The model under review builds one solid part; all positions refer to its coordinate system, in mm. A direction names the side the tool comes from. Give positions to 0.01 mm unless a question says otherwise; leave off trailing zeros. Write each loop counter-clockwise with the first axis right and the second up, starting at its lowest first coordinate (ties: lowest second). Pieces come first, ordered by that corner, then holes.
from build123d import *

# Parameters (mm, degrees)
SM_BASE_FLANGE_1_DEPTH = 2066
CUT_EXTRUDE_2_DEPTH    = 2.3
CUT_EXTRUDE_3_REACH    = 2082.296
CUT_EXTRUDE_4_REACH    = 2082.367
SKETCH_8_R             = 7


# Sheet-metal steps are written as plain solids
with BuildPart() as part:
    # Sketch 1 → Sm Base Flange 1 (new body)
    with BuildSketch(Plane.XY):
        with BuildLine():
            Line((33, 0), (3.3, 0))
            ThreePointArc((3.3, 0), (0.966547622, 0.966547622), (0, 3.3))
            Line((0, 3.3), (0, 52))
            ThreePointArc((0, 52), (0.966547622, 54.333452378), (3.3, 55.3))
            Line((3.3, 55.3), (22.085786438, 55.3))
            ThreePointArc((22.085786438, 55.3), (22.46846987, 55.376120467), (22.792893219, 55.592893219))
            Line((22.792893219, 55.592893219), (32.166547622, 64.966547622))
            ThreePointArc((32.166547622, 64.966547622), (34.5, 65.933095244), (36.833452378, 64.966547622))
            Line((36.833452378, 64.966547622), (46.207106781, 55.592893219))
            ThreePointArc((46.207106781, 55.592893219), (46.53153013, 55.376120467), (46.914213562, 55.3))
            Line((46.914213562, 55.3), (102.085786438, 55.3))
            ThreePointArc((102.085786438, 55.3), (102.46846987, 55.376120467), (102.792893219, 55.592893219))
            Line((102.792893219, 55.592893219), (112.166547622, 64.966547622))
            ThreePointArc((112.166547622, 64.966547622), (114.5, 65.933095244), (116.833452378, 64.966547622))
            Line((116.833452378, 64.966547622), (126.207106781, 55.592893219))
            ThreePointArc((126.207106781, 55.592893219), (126.53153013, 55.376120467), (126.914213562, 55.3))
            Line((126.914213562, 55.3), (182.085786438, 55.3))
            ThreePointArc((182.085786438, 55.3), (182.46846987, 55.376120467), (182.792893219, 55.592893219))
            Line((182.792893219, 55.592893219), (192.166547622, 64.966547622))
            ThreePointArc((192.166547622, 64.966547622), (194.5, 65.933095244), (196.833452378, 64.966547622))
            Line((196.833452378, 64.966547622), (206.207106781, 55.592893219))
            ThreePointArc((206.207106781, 55.592893219), (206.53153013, 55.376120467), (206.914213562, 55.3))
            Line((206.914213562, 55.3), (231.7, 55.3))
            ThreePointArc((231.7, 55.3), (234.033452378, 54.333452378), (235, 52))
            Line((235, 52), (235, 5.6))
            ThreePointArc((235, 5.6), (234.033452378, 3.266547622), (231.7, 2.3))
            Line((231.7, 2.3), (202, 2.3))
            Line((202, 2.3), (202, 4.6))
            Line((202, 4.6), (231.7, 4.6))
            ThreePointArc((231.7, 4.6), (232.407106781, 4.892893219), (232.7, 5.6))
            Line((232.7, 5.6), (232.7, 52))
            ThreePointArc((232.7, 52), (232.407106781, 52.707106781), (231.7, 53))
            Line((231.7, 53), (206.914213562, 53))
            ThreePointArc((206.914213562, 53), (205.651358236, 53.251197543), (204.580761184, 53.966547622))
            Line((204.580761184, 53.966547622), (195.207106781, 63.340202025))
            ThreePointArc((195.207106781, 63.340202025), (194.5, 63.633095244), (193.792893219, 63.340202025))
            Line((193.792893219, 63.340202025), (184.419238816, 53.966547622))
            ThreePointArc((184.419238816, 53.966547622), (183.348641764, 53.251197543), (182.085786438, 53))
            Line((182.085786438, 53), (126.914213562, 53))
            ThreePointArc((126.914213562, 53), (125.651358236, 53.251197543), (124.580761184, 53.966547622))
            Line((124.580761184, 53.966547622), (115.207106781, 63.340202025))
            ThreePointArc((115.207106781, 63.340202025), (114.5, 63.633095244), (113.792893219, 63.340202025))
            Line((113.792893219, 63.340202025), (104.419238816, 53.966547622))
            ThreePointArc((104.419238816, 53.966547622), (103.348641764, 53.251197543), (102.085786438, 53))
            Line((102.085786438, 53), (46.914213562, 53))
            ThreePointArc((46.914213562, 53), (45.651358236, 53.251197543), (44.580761184, 53.966547622))
            Line((44.580761184, 53.966547622), (35.207106781, 63.340202025))
            ThreePointArc((35.207106781, 63.340202025), (34.5, 63.633095244), (33.792893219, 63.340202025))
            Line((33.792893219, 63.340202025), (24.419238816, 53.966547622))
            ThreePointArc((24.419238816, 53.966547622), (23.348641764, 53.251197543), (22.085786438, 53))
            Line((22.085786438, 53), (3.3, 53))
            ThreePointArc((3.3, 53), (2.592893219, 52.707106781), (2.3, 52))
            Line((2.3, 52), (2.3, 3.3))
            ThreePointArc((2.3, 3.3), (2.592893219, 2.592893219), (3.3, 2.3))
            Line((3.3, 2.3), (33, 2.3))
            Line((33, 2.3), (33, 0))
        make_face()
    extrude(amount=SM_BASE_FLANGE_1_DEPTH)

    # Sketch 6 → Cut-Extrude 2 (cut)
    with BuildSketch(Plane.XZ.offset(-2.3)):
        with BuildLine():
            Line((213.5, 2055.5), (213.5, 2045.5))
            ThreePointArc((213.5, 2045.5), (219, 2040), (224.5, 2045.5))
            Line((224.5, 2045.5), (224.5, 2055.5))
            ThreePointArc((224.5, 2055.5), (219, 2061), (213.5, 2055.5))
        make_face()
    cut_extrude_2 = extrude(amount=-CUT_EXTRUDE_2_DEPTH, mode=Mode.SUBTRACT)

    # Sketch 7 → Cut-Extrude 3 (cut, up to next)
    with BuildSketch(Plane(origin=(0, 2.3, 0), x_dir=(-1, 0, 0), z_dir=(0, 1, 0)), mode=Mode.PRIVATE) as cut_extrude_3_sk1:
        with BuildLine():
            Line((-23.5, 2055.5), (-23.5, 2045.5))
            ThreePointArc((-23.5, 2045.5), (-18, 2040), (-12.5, 2045.5))
            Line((-12.5, 2045.5), (-12.5, 2055.5))
            ThreePointArc((-12.5, 2055.5), (-18, 2061), (-23.5, 2055.5))
        make_face()
    cut_extrude_3_tool1 = extrude(cut_extrude_3_sk1.sketch, amount=-CUT_EXTRUDE_3_REACH, mode=Mode.PRIVATE) & part.part
    cut_extrude_3 = cut_extrude_3_tool1.solids().sort_by_distance((18, 2.3, 2050.5))[0]
    add(cut_extrude_3, mode=Mode.SUBTRACT)

    # Mirror 1: Cut-Extrude 2, Cut-Extrude 3 across plane
    add(cut_extrude_2.mirror(Plane(origin=(0, 0, 1033), x_dir=(1, 0, 0), z_dir=(0, 0, -1))), mode=Mode.SUBTRACT)
    add(cut_extrude_3.mirror(Plane(origin=(0, 0, 1033), x_dir=(1, 0, 0), z_dir=(0, 0, -1))), mode=Mode.SUBTRACT)

    # Cut-Extrude 4: up to this face of the body (flat: up to its plane)
    cut_extrude_4_end = Plane(part.part.faces().sort_by_distance((0, 27.65, 1033))[0])
    # Sketch 8 → Cut-Extrude 4 (cut, up to the picked face)
    with BuildSketch(Plane(origin=(235, 0, 0), x_dir=(0, 0, -1), z_dir=(1, 0, 0)), mode=Mode.PRIVATE) as cut_extrude_4_sk1:
        with Locations((-2036, 30.3)):
            Circle(SKETCH_8_R)
    cut_extrude_4_tool1 = split(extrude(cut_extrude_4_sk1.sketch, amount=-CUT_EXTRUDE_4_REACH, mode=Mode.PRIVATE), bisect_by=cut_extrude_4_end, keep=Keep.BOTH, mode=Mode.PRIVATE)
    # Sketch 8 → Cut-Extrude 4 (cut, up to the picked face)
    with BuildSketch(Plane(origin=(235, 0, 0), x_dir=(0, 0, -1), z_dir=(1, 0, 0)), mode=Mode.PRIVATE) as cut_extrude_4_sk2:
        with Locations((-1986, 30.3)):
            Circle(SKETCH_8_R)
    cut_extrude_4_tool2 = split(extrude(cut_extrude_4_sk2.sketch, amount=-CUT_EXTRUDE_4_REACH, mode=Mode.PRIVATE), bisect_by=cut_extrude_4_end, keep=Keep.BOTH, mode=Mode.PRIVATE)
    # Sketch 8 → Cut-Extrude 4 (cut, up to the picked face)
    with BuildSketch(Plane(origin=(235, 0, 0), x_dir=(0, 0, -1), z_dir=(1, 0, 0)), mode=Mode.PRIVATE) as cut_extrude_4_sk3:
        with Locations((-1936, 30.3)):
            Circle(SKETCH_8_R)
    cut_extrude_4_tool3 = split(extrude(cut_extrude_4_sk3.sketch, amount=-CUT_EXTRUDE_4_REACH, mode=Mode.PRIVATE), bisect_by=cut_extrude_4_end, keep=Keep.BOTH, mode=Mode.PRIVATE)
    cut_extrude_4_1 = cut_extrude_4_tool1.solids().sort_by(Axis((235, 30.3, 2036), (-1, 0, 0)))[0]
    add(cut_extrude_4_1, mode=Mode.SUBTRACT)
    cut_extrude_4_2 = cut_extrude_4_tool2.solids().sort_by(Axis((235, 30.3, 1986), (-1, 0, 0)))[0]
    add(cut_extrude_4_2, mode=Mode.SUBTRACT)
    cut_extrude_4_3 = cut_extrude_4_tool3.solids().sort_by(Axis((235, 30.3, 1936), (-1, 0, 0)))[0]
    add(cut_extrude_4_3, mode=Mode.SUBTRACT)
    cut_extrude_4 = cut_extrude_4_1 + cut_extrude_4_2 + cut_extrude_4_3  # Cut-Extrude 4 as one shape, for the pattern or mirror that repeats it

    # Mirror 2: Cut-Extrude 4 across plane
    add(cut_extrude_4.mirror(Plane(origin=(0, 0, 1033), x_dir=(1, 0, 0), z_dir=(0, 0, -1))), mode=Mode.SUBTRACT)


solid = part.part
1) Consider section A-A, the plane x = 147.5. Give the boundary of the cut face in (y, z), then the cut area to 3 significant figures.
2) Tool access review of faces 4 (the flat face through (155, 53, 1019)), 5 (the flat face through (74, 55.3, 1019)), 6 (the flat face through (2.3, 28, 1019)): name each direction out of +Z, -Z, +X, -X, +Y, -Y from which nothing blocks a thin tool from reaching the whole face with its end or side.
3) Insertion check: pin 1 (2.5 mm diameter, centred on y = 1.5, z = 17.5, fed in from +X); pin 2 (8.5 mm diameter, centred on y = 30.3, z = 1986, fed in from +X); pin 3 (0.7 mm diameter, centred on y = 3.5, z = 2050, fed in from +X); pin 4 (1.5 mm diameter, centred on x = 79, z = 1144, fed in from -Y). Each pin has a flat end and moves straight along its axis. Give the tip position at first contact, or say it passes through.
4) The part is to be moulded in two halves that separate along Y. For faces 1 (the flat face through (75, 53, 1019)), 2 (the flat face through (232.7, 28, 1019)), 3 (the flat face through (0, 27, 1019)), say which applies: +Y half, -Y half, draft (parallel to the pull), parting line (faces both ways), or undercut.
5) To check wall thickness, follow probe 1 along X at (y, z) = (24.5, 682); probe 2 along X at (y, z) = (63, 490); probe 3 along Y at (x, z) = (234, 30). State the ranges of each line that lie inside material, in increasing order.
Answer block:
1. outline: (53, 0) - (55.3, 0) - (55.3, 2066) - (53, 2066) - close
1. area: 4,750 mm2
2. face 4: +Z, -Z, -Y
2. face 5: +Z, -Z, +Y
2. face 6: +Z, -Z
3. pin 1: stops at x = 233.36
3. pin 2: passes through
3. pin 3: stops at x = 234.5
3. pin 4: stops at y = 53
4. face 1: -Y half
4. face 2: undercut
4. face 3: draft
5. probe 1: x = 0 to 2.3, 232.7 to 235
5. probe 2: x = 30.2 to 33.45, 35.55 to 38.8, 110.2 to 113.45, 115.55 to 118.8, 190.2 to 193.45, 195.55 to 198.8
5. probe 3: y = 3.23 to 23.3, 37.3 to 54.37
